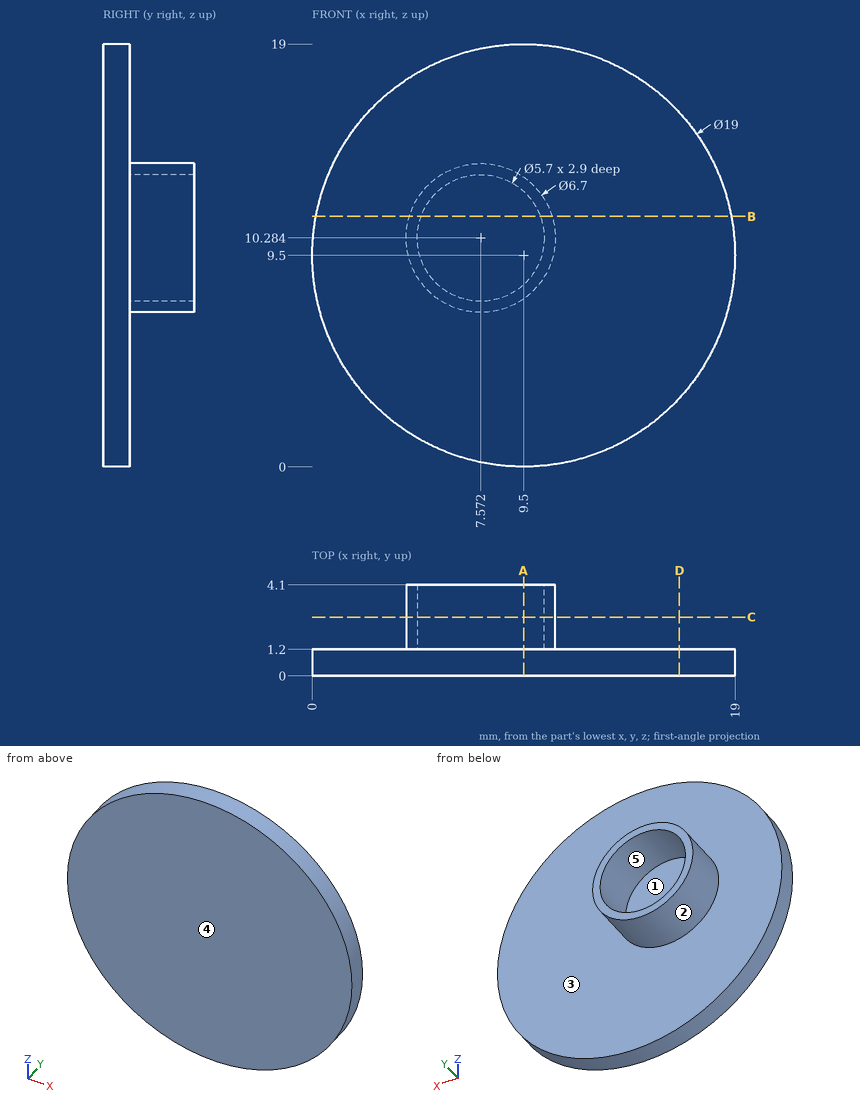
Study the drawing (mm; zero at the part's minimum x, y, z) and answer. A direction names the side the tool comes from. Coordinates: 2 decimals unless noted, no trailing zeros. Loops run counter-clockwise (first coordinate to the right, second up) from the corner with the lowest first, then second, coordinate; pieces in that order, holes last. Notation, with made-up numbers: (-5, 14) -> (23, 14) arc R10 cw to (23, 19) -> close; hole circle Ø6 at (31, -23). An arc over 180 degrees is marked (long way). Answer in a Markdown table with one row per item. Add a question column.
1. The part is cut by section B-B, the plane z = 11.25. Write down the section's boundary in (x, y).
2. The part is cut by section C-C, the plane y = 2.65. Write down the section's boundary in (x, z).
3. For the marked faces 4 and 5, determine the directions among +Z, -Z, +X, -X, +Y, -Y from which every point of the face is accessible in a straight line to the end or side of a thin tool.
4. Consider line 1 (Y direction, x = 8, z = 2.25); line 2 (Z direction, x = 10, y = 2.45) (1 decimal); line 3 (X direction, y = 3.2, z = 11) (1 decimal). Determine where each line is inside the solid, lowest interval first. Write a range as [from, to].
5. The part is cut by section A-A, the plane x = 9.5. Write down the section's boundary in (y, z) (1 decimal).
6. Flat-ended cylindrical pins translate along their axes: P1, Ø1, axis at x = 10.5, z = 4, coming from the +Y side; P2, Ø2, axis at y = 1, z = 2.5, coming from the -X side (1 decimal). Find the tip coordinate at first contact, or state that the pin passes through.
7. The part is cut by section D-D, the plane x = 16.5. Write down the section's boundary in (y, z), then the cut area to 3 significant figures.
8. Determine the mould class of the marked faces 1, 2 and 3 for opening direction X: +X half, -X half, draft (parallel to the pull), parting line (faces both ways), or undercut.
Answer below:
| question | item | result |
|---|---|---|
| 1 | outline | (0.16, 0) -> (18.84, 0) -> (18.84, 1.2) -> (10.78, 1.2) -> (10.78, 4.1) -> (10.25, 4.1) -> (10.25, 1.2) -> (4.89, 1.2) -> (4.89, 4.1) -> (4.36, 4.1) -> (4.36, 1.2) -> (0.16, 1.2) -> close |
| 2 | outline | circle Ø6.7 at (7.57, 10.28); hole circle Ø5.7 at (7.57, 10.28) |
| 3 | face 4 | +Z, -Z, +X, -X, -Y |
| 3 | face 5 | +Y |
| 4 | line 1 | [0, 1.2] |
| 4 | line 2 | [8, 8.8], [11.8, 12.6] |
| 4 | line 3 | [4.3, 4.8], [10.3, 10.8] |
| 5 | outline | (0, 0) -> (1.2, 0) -> (1.2, 7.5) -> (4.1, 7.5) -> (4.1, 8.2) -> (1.2, 8.2) -> (1.2, 12.4) -> (4.1, 12.4) -> (4.1, 13) -> (1.2, 13) -> (1.2, 19) -> (0, 19) -> close |
| 6 | P1 | y = 1.2 |
| 6 | P2 | x = 2.1 |
| 7 | outline | (0, 3.08) -> (1.2, 3.08) -> (1.2, 15.92) -> (0, 15.92) -> close |
| 7 | area | 15.4 mm2 |
| 8 | face 1 | undercut |
| 8 | face 2 | parting line |
| 8 | face 3 | draft |
